Design review of the part built by this model. Coordinates are the model's own, in mm. Face numbers are marked on the shaded views. Round coordinates to 2 decimals unless told otherwise and drop trailing zeros. Order: outer loops, then holes, each group sorted by start corner. A loop starts at its lowest first (then second) coordinate and runs counter-clockwise, first axis right, second up. Notation, with made-up numbers: (36.5, -7.5) - (47.5, -7.5) arc R30 cw to (47.5, 19.5) - close; hole circle Ø5 at (10, 61). An arc over 180 degrees is marked (long way). Write item = value, one per line.
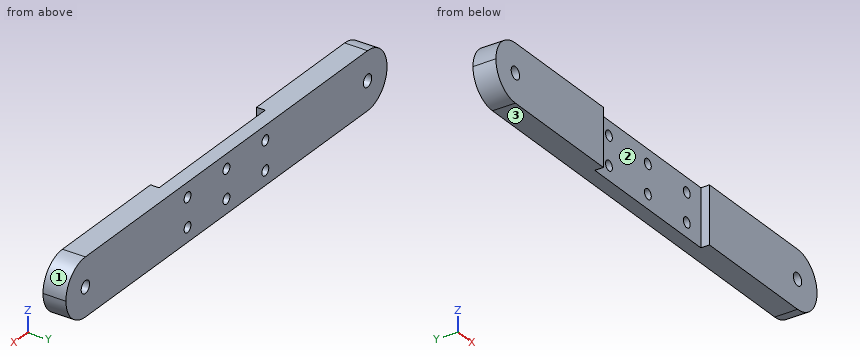
from build123d import *

# Parameters (mm, degrees)
EXTRUDE_1_DEPTH     = 20
SKETCH_2_R          = 2.15
SKETCH_2_R_2        = 1.75
CUT_EXTRUDE_1_DEPTH = 20
FILLET_1_R          = 10


with BuildPart() as part:
    # 스케치1 → 보스-돌출1 (new body)
    with BuildSketch(Plane.XY):
        Polygon((28, -2.5), (83.25, -2.5), (83.25, 5.5), (-81.75, 5.5), (-81.75, -2.5), (-26.5, -2.5), (-26.5, 0.5), (28, 0.5), align=None)
    extrude(amount=EXTRUDE_1_DEPTH)

    # 스케치2 → 컷-돌출1 (cut)
    with BuildSketch(Plane(origin=(0, 5.5, 0), x_dir=(1, 0, 0), z_dir=(0, 1, 0))):
        with Locations(Location((-71.75, -10, 0), (0, 0, 270))):
            Circle(SKETCH_2_R)
        with Locations(Location((73.25, -10, 0), (0, 0, 270))):
            Circle(SKETCH_2_R)
        with Locations(Location((-19.25, -5, 0), (0, 0, 270))):
            Circle(SKETCH_2_R_2)
        with Locations(Location((0.75, -5, 0), (0, 0, 270))):
            Circle(SKETCH_2_R_2)
        with Locations(Location((20.75, -5, 0), (0, 0, 270))):
            Circle(SKETCH_2_R_2)
        with Locations(Location((20.75, -15, 0), (0, 0, 270))):
            Circle(SKETCH_2_R_2)
        with Locations(Location((0.75, -15, 0), (0, 0, 270))):
            Circle(SKETCH_2_R_2)
        with Locations(Location((-19.25, -15, 0), (0, 0, 270))):
            Circle(SKETCH_2_R_2)
    extrude(amount=-CUT_EXTRUDE_1_DEPTH, mode=Mode.SUBTRACT)

    # 필렛1
    fillet_1_edges = [part.edges().sort_by_distance(p)[0] for p in [
        (83.25, 1.5, 0),
        (83.25, 1.5, 20),
        (-81.75, 1.5, 0),
        (-81.75, 1.5, 20),
    ]]
    fillet(fillet_1_edges, radius=FILLET_1_R - 0.0001)  # a hair under: the kernel refuses the full size


solid = part.part
1) To check wall thickness, follow L1, parallel to Z at x = 73, y = -1.5; L2, parallel to X at y = 4.1, z = 5; L3, parallel to X at y = 5, z = 6.5. State the ranges of each line that lie inside material, in increasing order. Write a range as from..to.
Findings:
L1 = 0..7.86, 12.14..20
L2 = -80.41..-21, -17.5..-1, 2.5..19, 22.5..81.91
L3 = -81.12..-20.15, -18.35..-0.15, 1.65..19.85, 21.65..82.62
2) The part is to be moulded in two halves that separate along X. For the marked faces 1, 2 and 3, say which applies: released by +X, released by -X, zero draft, split by the parting line, or undercut.
Findings:
face_1 = released by +X
face_2 = undercut
face_3 = zero draft
3) Clearance check with flat-ended pins moving along their axes: pin 1 Ø4.5 at (x, z) = (-19.25, 5) entering from -Y; pin 2 Ø3 at (y, z) = (3, 3.5) entering from +X; pin 3 Ø2.5 at (y, z) = (-1.5, 8.5) entering from +X; pin 4 Ø2.5 at (x, z) = (73.25, 10) entering from -Y. State where each tip first meets the part, or that it passes through.
Findings:
pin_1 = 0.5
pin_2 = 81.91
pin_3 = 83.25
pin_4 = through
4) We need section A-A on x = 0.75. Write out the cut boundary in (y, z), and give its area (3 significant figures).
Findings:
outline = (0.5, 0) - (5.5, 0) - (5.5, 3.25) - (0.5, 3.25) - close; (0.5, 6.75) - (5.5, 6.75) - (5.5, 13.25) - (0.5, 13.25) - close; (0.5, 16.75) - (5.5, 16.75) - (5.5, 20) - (0.5, 20) - close
area = 65.0 mm^2
5) We need section C-C on z = 15. Write out the cut boundary in (x, y), and give its area (3 significant figures).
Findings:
outline = (-80.41, -2.5) - (-26.5, -2.5) - (-26.5, 0.5) - (-21, 0.5) - (-21, 5.5) - (-80.41, 5.5) - close; (-17.5, 0.5) - (-1, 0.5) - (-1, 5.5) - (-17.5, 5.5) - close; (2.5, 0.5) - (19, 0.5) - (19, 5.5) - (2.5, 5.5) - close; (22.5, 0.5) - (28, 0.5) - (28, -2.5) - (81.91, -2.5) - (81.91, 5.5) - (22.5, 5.5) - close
area = 1,080 mm^2
6) We need section B-B on y = 3.75. Give the number of separate pieces and of enclosed holes in the cut face, and give its area (3 significant figures).
Findings:
separate_pieces = 1
enclosed_holes = 8
area = 3,130 mm^2
